```python
from build123d import *

# Parameters (mm, degrees)
SKETCH1_R               = 12.7
BOSS_EXTRUDE1_DEPTH     = 1
CUT_EXTRUDE1_DEPTH      = 18.98832955
CUT_EXTRUDE1_DEPTH_BACK = 18.98832955
SKETCH19_R              = 1
CUT_EXTRUDE2_DEPTH      = 18.98832955
CUT_EXTRUDE2_DEPTH_BACK = 18.98832955
SKETCH20_R              = 7.5
SKETCH21_W              = 65.874202484
SKETCH21_H              = 51.979273979
CUT_EXTRUDE3_DEPTH      = 18.98832955
CUT_EXTRUDE4_DEPTH      = 18.98832955
CUT_EXTRUDE4_DEPTH_BACK = 18.98832955
SKETCH22_R              = 1


with BuildPart() as part:
    # Sketch1 → Boss-Extrude1 (new body)
    with BuildSketch(Plane(origin=(0, 0, 0), x_dir=(1, 0, 0), z_dir=(0, 1, 0))):
        with Locations(Location((0, 0, 0), (0, 0, 270))):
            Circle(SKETCH1_R)
    extrude(amount=BOSS_EXTRUDE1_DEPTH)

    # Sketch19 → Cut-Extrude1 (cut, two sides: drawn at the far end of the back side and taken through both)
    with BuildSketch(Plane(origin=(0, 1, 0), x_dir=(1, 0, 0), z_dir=(0, 1, 0)).offset(-CUT_EXTRUDE1_DEPTH_BACK)):
        with Locations(Location((0, 11, 0), (0, 0, 270))):
            Circle(SKETCH19_R)
        with Locations(Location((9.526279442, 5.5, 0), (0, 0, 270))):
            Circle(SKETCH19_R)
        with Locations(Location((9.526279442, -5.5, 0), (0, 0, 270))):
            Circle(SKETCH19_R)
        with Locations(Location((0, -11, 0), (0, 0, 270))):
            Circle(SKETCH19_R)
        with Locations(Location((-9.526279442, -5.5, 0), (0, 0, 270))):
            Circle(SKETCH19_R)
        with Locations(Location((-9.526279442, 5.5, 0), (0, 0, 270))):
            Circle(SKETCH19_R)
    extrude(amount=CUT_EXTRUDE1_DEPTH + CUT_EXTRUDE1_DEPTH_BACK, mode=Mode.SUBTRACT)

    # Sketch20 → Cut-Extrude2 (cut, two sides: drawn at the far end of the back side and taken through both)
    with BuildSketch(Plane(origin=(0, 1, 0), x_dir=(1, 0, 0), z_dir=(0, 1, 0)).offset(-CUT_EXTRUDE2_DEPTH_BACK)):
        with Locations(Location((0, 0, 0), (0, 0, 270))):
            Circle(SKETCH20_R)
    extrude(amount=CUT_EXTRUDE2_DEPTH + CUT_EXTRUDE2_DEPTH_BACK, mode=Mode.SUBTRACT)

    # Sketch21 → Cut-Extrude3 (cut, through all)
    with BuildSketch(Plane.XY):
        with Locations((-3.816154381, 6.321647006)):
            Rectangle(SKETCH21_W, SKETCH21_H)
    extrude(amount=-CUT_EXTRUDE3_DEPTH, mode=Mode.SUBTRACT)

    # Sketch22 → Cut-Extrude4 (cut, two sides: drawn at the far end of the back side and taken through both)
    with BuildSketch(Plane(origin=(0, 1, 0), x_dir=(1, 0, 0), z_dir=(0, 1, 0)).offset(-CUT_EXTRUDE4_DEPTH_BACK)):
        with Locations(Location((-2.847009496, -10.625184089, 0), (0, 0, 270))):
            Circle(SKETCH22_R)
    extrude(amount=CUT_EXTRUDE4_DEPTH + CUT_EXTRUDE4_DEPTH_BACK, mode=Mode.SUBTRACT)


solid = part.part
```
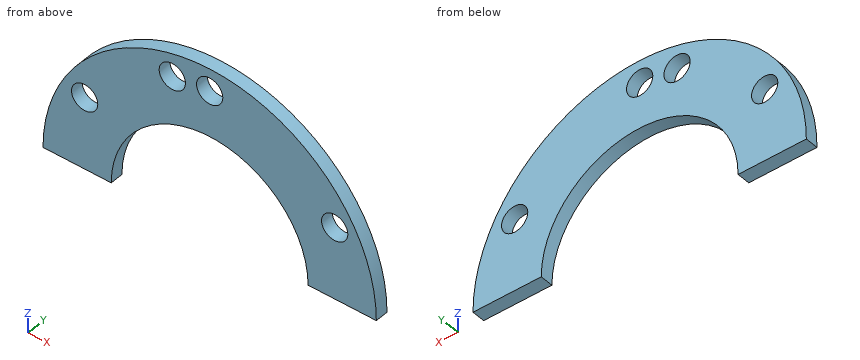
For this review, take the finished solid that the model builds, in its own axes (mm). Give positions to 0.01 mm unless a question says otherwise; leave off trailing zeros. Write each loop counter-clockwise with the first axis right and the second up, starting at its lowest first coordinate (ties: lowest second). Pieces come first, ordered by that corner, then holes. Notation, with made-up numbers: M 28.5,85.5 L 42.5,85.5 A21 ccw 42.5,93.5 Z; hole C -14,-31 d10. An arc over 180 degrees is marked long. One line per item, written item: value.
1) Take a section at D-D, the plane y = 0.3. Write out the cut boundary in (x, z).
Results are:
outline: M -12.7,0 L -7.5,0 A7.5 cw 7.5,0 L 12.7,0 A12.7 ccw Z; hole C -9.53,5.5 d2; hole C -2.85,10.63 d2; hole C 0,11 d2; hole C 9.53,5.5 d2
2) Take a section at A-A, the plane x = 0. Write out the cut boundary in (y, z).
Results are:
outline: M 0,7.5 L 1,7.5 L 1,10 L 0,10 Z; M 0,12 L 1,12 L 1,12.7 L 0,12.7 Z
3) For line 1 (X direction, y = 0.5, z = 5.5); line 2 (Z direction, x = 0, y = 0.75); line 3 (X direction, y = 0.7, z = 11), list the stretches that pass through material, from the lowest coordinate up. Write a range as from..to.
Results are:
line 1: x = -11.45..-10.53, -8.53..-5.1, 5.1..8.53, 10.53..11.45
line 2: z = 7.5..10, 12..12.7
line 3: x = -6.35..-3.77, -1.92..-1, 1..6.35
4) Take a section at B-B, the plane z = 11. Write out the cut boundary in (x, y), then the cut area to 3 significant figures.
Results are:
outline: M -6.35,0 L -3.77,0 L -3.77,1 L -6.35,1 Z; M -1.92,0 L -1,0 L -1,1 L -1.92,1 Z; M 1,0 L 6.35,0 L 6.35,1 L 1,1 Z
area: 8.84 mm²
5) For P1, Ø1.8, axis at x = 9.53, z = 5.5, coming from the -Y side, flat-tipped, find the tip position at first contact; note if it passes through.
Results are:
P1: passes through
6) Take a section at C-C, the plane z = 3.25. Write out the cut boundary in (x, y).
Results are:
outline: M -12.28,0 L -6.76,0 L -6.76,1 L -12.28,1 Z; M 6.76,0 L 12.28,0 L 12.28,1 L 6.76,1 Z
